from build123d import *

# Parameters (mm, degrees)
F0_W     = 120
F0_H     = 16
F1_DEPTH = 3
F2_R     = 4.6
F3_DEPTH = 100


with BuildPart() as f1:
    # F0 (on Top) → F1 (new body)
    with BuildSketch(Plane.XY):
        Rectangle(F0_W, F0_H)
    extrude(amount=F1_DEPTH)

    # F2 (on Top) → F3 (join)
    with BuildSketch(Plane.XY):
        with Locations((-45, 0)):
            Circle(F2_R)
        with Locations((45, 0)):
            Circle(F2_R)
    extrude(amount=F3_DEPTH)


solid = f1.part
Geometry check sheet. Reference: the model listing, model coordinates, mm. A direction names the side the tool comes from. Round coordinates to 2 decimals unless told otherwise and drop trailing zeros. Write each loop counter-clockwise with the first axis right and the second up, starting at its lowest first coordinate (ties: lowest second). Pieces come first, ordered by that corner, then holes. Notation, with made-up numbers: (-4.5, 20) - (14.5, 20) arc R10 cw to (14.5, 31) - close; hole circle Ø11 at (-17, 88.25). An arc over 180 degrees is marked (long way). One line per item, written item: value.
1. Cross-section at B-B on x = -45. Record the boundary of the cut face in (y, z).
The answers:
outline: (-8, 0) - (8, 0) - (8, 3) - (4.6, 3) - (4.6, 100) - (-4.6, 100) - (-4.6, 3) - (-8, 3) - close
2. Cross-section at A-A on y = 0. Record the boundary of the cut face in (x, z).
The answers:
outline: (-60, 0) - (60, 0) - (60, 3) - (49.6, 3) - (49.6, 100) - (40.4, 100) - (40.4, 3) - (-40.4, 3) - (-40.4, 100) - (-49.6, 100) - (-49.6, 3) - (-60, 3) - close
3. Cross-section at D-D on y = -6.5. Record the boundary of the cut face in (x, z), and give its area (3 significant figures).
The answers:
outline: (-60, 0) - (60, 0) - (60, 3) - (-60, 3) - close
area: 360 mm^2
4. Mould release check, pull along X, two halves, no side actions. Record for faces 3 (the face through (-45, 0, 100)), 4 (the face through (-1, 0, 3)), 5 (the face through (-40.61, 1.38, 50.82)), 6 (the face through (-60, 0, 1)): released by +X, released by -X, zero draft, split by the parting line, or undercut.
The answers:
face 3: zero draft
face 4: undercut
face 5: undercut
face 6: released by -X
5. Set-up check for faces 1 (the face through (45, 0, 100)), 2 (the face through (49.39, 1.38, 50.82)): record each of +Z, -Z, +X, -X, +Y, -Y from which the full face is reachable in a straight line by a thin tool's end or side.
The answers:
face 1: +Z, +X, -X, +Y, -Y
face 2: +Z
6. Cross-section at C-C on z = 80. Record the boundary of the cut face in (x, y).
The answers:
outline: circle Ø9.2 at (-45, 0); circle Ø9.2 at (45, 0)
7. Scan lines: L1, parallel to Z at x = 18, y = 1.25; L2, parallel to Y at x = -44.5, z = 94.5; L3, parallel to X at y = -2, z = 33. Record each from-to range of solid material in increasing order.
The answers:
L1: z = 0 to 3
L2: y = -4.57 to 4.57
L3: x = -49.14 to -40.86, 40.86 to 49.14
8. Depth check by flat-ended pin: pin 1 Ø5 at (x, y) = (-20.5, -2) entering from +Z; pin 2 Ø5 at (y, z) = (-2.5, 65) entering from -X; pin 3 Ø6 at (x, z) = (45, 17.5) entering from +Y. Enter the tip coordinate at first touch or a pass-through.
The answers:
pin 1: stops at z = 3
pin 2: stops at x = -49.6
pin 3: stops at y = 4.6
